from build123d import *

# Parameters (mm, degrees)
F1_DEPTH = 50.8
F2_T     = -2.54


with BuildPart() as f1:
    # F0 (on Top) → F1 (new body)
    with BuildSketch(Plane.XY):
        with BuildLine():
            Line((71.33154, 17.38706), (-72.223172, 17.38706))
            ThreePointArc((-72.223172, 17.38706), (-98.990059, -16.495419), (-72.223172, -50.377898))
            Line((-72.223172, -50.377898), (71.33154, -50.377898))
            Line((71.33154, -50.377898), (71.33154, 17.38706))
        make_face()
    extrude(amount=F1_DEPTH)

    # F2
    f2_openings = [f1.faces().sort_by_distance(p)[0] for p in [
        (-10.546065, -16.495419, 50.8),
    ]]
    offset(amount=F2_T, openings=f2_openings)


solid = f1.part
Work out the finished part from the listing and answer in its coordinate system (mm). A direction names the side the tool comes from. Give positions to 0.01 mm unless a question says otherwise; leave off trailing zeros. Order: outer loops, then holes, each group sorted by start corner. A loop starts at its lowest first (then second) coordinate and runs counter-clockwise, first axis right, second up. Notation, with made-up numbers: (62, 76.25) - (98, 76.25) arc R21 cw to (98, 99.25) - close; hole circle Ø1 at (21.5, 39.25). An arc over 180 degrees is marked (long way). Answer as CSV lines item,"result". Start each with the question number.
Q1. The mould has two halves that part along X. Classify faces 3 (the face through (-15, -16, 0)), 4 (the face through (-3, -47.838, 26)), 5 (the face through (71.332, -17, 25)): +X half, -X half, draft (parallel to the pull), parting line (faces both ways), or undercut.
Q2. For faces 1 (the face through (-96.444, -15.895, 26.332)), 2 (the face through (-98.984, -15.843, 25.044)), determine the directions among +Z, -Z, +X, -X, +Y, -Y from which every point of the face is accessible in a straight line to the end or side of a thin tool.
Q3. The part is cut by section B-B (x = 56.5). Write down the section's boundary in (y, z).
Q4. The part is cut by section C-C (y = -11). Write down the section's boundary in (x, z).
Q5. Find the intervals of material crossed by L1, parallel to Y at x = 56, z = 22.5; L2, parallel to X at y = -17, z = 7.5; L3, parallel to Z at x = 30, y = 10.5, in increasing order. Write a range as [from, to].
Q6. Given pin 1 Ø5 at (x, y) = (-75, -11.5) entering from +Z; pin 2 Ø1 at (x, y) = (-24, -0.5) entering from -Z; pin 3 Ø1 at (y, z) = (8.5, 18.5) entering from -X, each flat-ended and moving along its own axis, determine where each tip first touches the part or whether it passes through.
Q7. The part is cut by section A-A (z = 21). Write down the section's boundary in (x, y).
Check result:
1,face 3,"draft"
1,face 4,"undercut"
1,face 5,"+X half"
2,face 1,"+Z"
2,face 2,"+Z, -Z, -X"
3,outline,"(-50.38, 0) - (17.39, 0) - (17.39, 50.8) - (14.85, 50.8) - (14.85, 2.54) - (-47.84, 2.54) - (-47.84, 50.8) - (-50.38, 50.8) - close"
4,outline,"(-98.55, 0) - (71.33, 0) - (71.33, 50.8) - (68.79, 50.8) - (68.79, 2.54) - (-95.98, 2.54) - (-95.98, 50.8) - (-98.55, 50.8) - close"
5,L1,"y = [-50.38, -47.84], [14.85, 17.39]"
5,L2,"x = [-98.99, -96.45], [68.79, 71.33]"
5,L3,"z = [0, 2.54]"
6,pin 1,"stops at z = 2.54"
6,pin 2,"stops at z = 0"
6,pin 3,"stops at x = -88.92"
7,outline,"(-72.22, -50.38) - (71.33, -50.38) - (71.33, 17.39) - (-72.22, 17.39) arc R34.83 ccw to start; hole (-71.92, -47.84) - (68.79, -47.84) - (68.79, 14.85) - (-71.92, 14.85) arc R32.29 ccw to start"
